Could you check a few things on this model? Use its own coordinates, in mm. A direction names the side the tool comes from. Coordinates: 2 decimals unless noted, no trailing zeros. Order: outer loops, then holes, each group sorted by start corner. A loop starts at its lowest first (then second) coordinate and runs counter-clockwise, first axis right, second up.
```python
from build123d import *

# Parameters (mm, degrees)
SKETCH_5_R          = 1.6
CUT_EXTRUDE_1_DEPTH = 5
SKETCH_6_R          = 1.6
CUT_EXTRUDE_2_DEPTH = 5
SKETCH_7_R          = 3.5
EXTRUDE_1_DEPTH     = 1


with BuildPart() as part:
    # 草图4 → 旋转1 (revolve)
    with BuildSketch(Plane.XY, mode=Mode.PRIVATE) as revolve_1_sk:
        Polygon((0, 30.5), (-18, 30.5), (-21, 27.5), (-21, 1.5), (-10, 1.5), (-10, 0), (0, 0), align=None)
    revolve(revolve_1_sk.sketch.rotate(Axis((0, 0, 0), (0, 1, 0)), 180), axis=Axis((0, 0, 0), (0, 1, 0)))

    # 草图5 → 切除-拉伸1 (cut)
    with BuildSketch(Plane(origin=(0, 30.5, 0), x_dir=(1, 0, 0), z_dir=(0, 1, 0))):
        with Locations(Location((0, 8, 0), (0, 0, 270))):
            Circle(SKETCH_5_R)
        with Locations(Location((6.92820323, 4, 0), (0, 0, 270))):
            Circle(SKETCH_5_R)
        with Locations(Location((6.92820323, -4, 0), (0, 0, 270))):
            Circle(SKETCH_5_R)
        with Locations(Location((0, -8, 0), (0, 0, 270))):
            Circle(SKETCH_5_R)
        with Locations(Location((-6.92820323, -4, 0), (0, 0, 270))):
            Circle(SKETCH_5_R)
        with Locations(Location((-6.92820323, 4, 0), (0, 0, 270))):
            Circle(SKETCH_5_R)
    extrude(amount=-CUT_EXTRUDE_1_DEPTH, mode=Mode.SUBTRACT)

    # 草图6 → 切除-拉伸2 (cut)
    with BuildSketch(Plane.XZ.offset(-1.5)):
        with Locations(Location((0, 18, 0), (0, 0, 270))):
            Circle(SKETCH_6_R)
        with Locations(Location((18, 0, 0), (0, 0, 270))):
            Circle(SKETCH_6_R)
        with Locations(Location((0, -18, 0), (0, 0, 270))):
            Circle(SKETCH_6_R)
        with Locations(Location((-18, 0, 0), (0, 0, 270))):
            Circle(SKETCH_6_R)
    extrude(amount=-CUT_EXTRUDE_2_DEPTH, mode=Mode.SUBTRACT)

    # 草图7 → 凸台-拉伸1 (add)
    with BuildSketch(Plane(origin=(0, 30.5, 0), x_dir=(1, 0, 0), z_dir=(0, 1, 0))):
        Circle(SKETCH_7_R)
    extrude(amount=EXTRUDE_1_DEPTH)


solid = part.part
```
Item 1: I need wall thicknesses on line 1 (X direction, y = 27, z = 4); line 2 (Y direction, x = 9, z = 12.5); line 3 (Y direction, x = 4, z = 1.5). Which ranges of each line are inside material? Lowest first, please.
Item 2: Thinking about a two-plate mould opening in X: for faces 4 (the face through (9, 1.5, -5)), 5 (the face through (0, 6.5, -18)), 6 (the face through (-3.94, 30.31, 17.76)), which applies, +X half, -X half, draft (parallel to the pull), parting line (faces both ways), or undercut?
Item 3: Suppose I cut it at B-B (y = 5.5). List the corners of the cut face in (x, z) for me.
Item 4: Which directions (+Z, -Z, +X, -X, +Y, -Y) give clear straight access to the entire face, cutting with the end or side of a thin tool? Please do faces 1 (the face through (0, 25.5, -8)), 2 (the face through (20.03, 14.32, -6.31)), 3 (the face through (0.07, 3.96, 19.6)).
Item 5: For pin 1 Ø1.5 at (x, z) = (-15, -6.5) entering from +Y; pin 2 Ø2 at (y, z) = (18, -12.5) entering from -X; pin 3 Ø8 at (x, y) = (11, 23) entering from +Z, each with a flat end and sliding along its axis, tell me the tip position at first contact or that it passes through.
Geometry results:
1. line 1: x = -20.62 to -8.53, -5.33 to 5.33, 8.53 to 20.62
1. line 2: y = 1.5 to 30.5
1. line 3: y = 0 to 30.5
2. face 4: draft
2. face 5: undercut
2. face 6: parting line
3. outline: circle Ø42 at (0, 0); hole circle Ø3.2 at (-18, 0); hole circle Ø3.2 at (0, -18); hole circle Ø3.2 at (0, 18); hole circle Ø3.2 at (18, 0)
4. face 1: +Y
4. face 2: +Y, -Y
4. face 3: -Y
5. pin 1: stops at y = 30.5
5. pin 2: stops at x = -17.57
5. pin 3: stops at z = 19.8
